from build123d import *

# Parameters (mm, degrees)
SKETCH1_R           = 50
BOSS_EXTRUDE1_DEPTH = 20
SKETCH2_W           = 20
SKETCH2_H           = 75
BOSS_EXTRUDE2_DEPTH = 65
SKETCH3_R           = 7.5
CUT_EXTRUDE1_DEPTH  = 65
FILLET1_R           = 37.5
SKETCH4_R           = 41.355609665
BOSS_EXTRUDE3_DEPTH = 35
SKETCH8_R           = 15
CUT_EXTRUDE2_DEPTH  = 20
SKETCH10_W          = 5
SKETCH10_H          = 8.446283525


with BuildPart() as part:
    # Sketch1 → Boss-Extrude1 (new body)
    with BuildSketch(Plane.XY):
        Circle(SKETCH1_R)
    extrude(amount=BOSS_EXTRUDE1_DEPTH)

    # Sketch2 → Boss-Extrude2 (add)
    with BuildSketch(Plane(origin=(0, 0, 0), x_dir=(-1, 0, 0), z_dir=(0, 0, -1))):
        Rectangle(SKETCH2_W, SKETCH2_H)
    extrude(amount=BOSS_EXTRUDE2_DEPTH)

    # Sketch3 → Cut-Extrude1 (cut)
    with BuildSketch(Plane(origin=(10, 0, 0), x_dir=(0, 0, -1), z_dir=(1, 0, 0))):
        with Locations((39.996807152, 0)):
            Circle(SKETCH3_R)
    extrude(amount=-CUT_EXTRUDE1_DEPTH, mode=Mode.SUBTRACT)

    # Fillet1
    fillet1_edges = [part.edges().sort_by_distance(p)[0] for p in [
        (0, -37.5, -65),
        (0, 37.5, -65),
    ]]
    fillet(fillet1_edges, radius=FILLET1_R - 0.0001)  # a hair under: the kernel refuses the full size

    # Sketch4 → Boss-Extrude3 (add)
    with BuildSketch(Plane.XY.offset(20)):
        Circle(SKETCH4_R)
    extrude(amount=BOSS_EXTRUDE3_DEPTH)

    # Sketch8 → Cut-Extrude2 (cut)
    with BuildSketch(Plane.XY.offset(55)):
        Circle(SKETCH8_R)
    extrude(amount=-CUT_EXTRUDE2_DEPTH, mode=Mode.SUBTRACT)

    # Sketch10 → Cut-Revolve1 (revolve, cut)
    with BuildSketch(Plane(origin=(0, 0, 0), x_dir=(0, 0, -1), z_dir=(1, 0, 0)), mode=Mode.PRIVATE) as cut_revolve1_sk:
        with Locations((-37.5, 15.776858238)):
            Rectangle(SKETCH10_W, SKETCH10_H)
    revolve(cut_revolve1_sk.sketch.rotate(Axis((0, 0, 55), (0, 0, -1)), 90), axis=Axis((0, 0, 55), (0, 0, -1)), mode=Mode.SUBTRACT)


solid = part.part
Geometry: final body of the model. Coordinates: model frame, mm. A direction names the side the tool comes from. Coordinates: 2 decimals unless noted, no trailing zeros. Loops run counter-clockwise (first coordinate to the right, second up) from the corner with the lowest first, then second, coordinate; pieces in that order, holes last. Notation, with made-up numbers: (45, -14) - (86, -14) arc R4 ccw to (86, -8) - close; hole circle Ø3 at (-34, -19.75). An arc over 180 degrees is marked (long way). Put each result on its own line as item: value. Start each with the question number.
Q1. Set-up query: faces 5 (the cylindrical face through (-14.985, 0.66, 47.605)), 6 (the flat face through (0, -37.5, -14)), 7 (the flat face through (0, 37.5, -14)), 8 (the flat face through (0, 0, 35)), 9 (the flat face through (10, -1, -32)). Return all of +Z, -Z, +X, -X, +Y, -Y with unobstructed straight access to the full face (end or side cutting, diameter ignored); none if empty.
Q2. Pull-direction query (Z, two-part tool) for faces 1 (the flat face through (-10, -1, -32)), 2 (the flat face through (-3, -15, 40)), 3 (the cylindrical face through (-0.14, -26.81, -53.72)), 4 (the flat face through (18, 1, 55)); classes: released by +Z, released by -Z, zero draft, split by the parting line, or undercut.
Q3. Line query: line 1 (Y direction, x = 0, z = 37); line 2 (Y direction, x = 0, z = 44); line 3 (Z direction, x = -17, y = -4.5). Output: solid intervals per line, ascending.
Q4. Pin query (flat end, axial travel): pin 1 Ø8 at (x, z) = (-11, 21) entering from +Y; pin 2 Ø19.5 at (y, z) = (0, -40) entering from -X; pin 3 Ø6 at (x, z) = (-2.5, -19.5) entering from +Y. Return the tip coordinate at first contact, or that it passes through.
Q5. Cut plane C-C, the plane y = 3. Return loops of the section in (x, z), and give its area (3 significant figures).
Q6. Cut plane D-D, the plane x = -33.5. Return loops of the section in (y, z).
Q7. Cut plane B-B, the plane z = 47. Return loops of the section in (x, y), and give its area (3 significant figures).
Filled sheet:
1. face 5: +Z
1. face 6: -Z, +X, -X, -Y
1. face 7: -Z, +X, -X, +Y
1. face 8: none
1. face 9: -Z, +X, +Y, -Y
2. face 1: zero draft
2. face 2: undercut
2. face 3: released by -Z
2. face 4: released by +Z
3. line 1: -41.36 to -20, 20 to 41.36
3. line 2: -41.36 to -15, 15 to 41.36
3. line 3: 0 to 35, 40 to 55
4. pin 1: y = 49.49
4. pin 2: x = -10
4. pin 3: y = 37.5
5. outline: (-49.91, 0) - (-10, 0) - (-10, -33.12) - (10, -33.12) - (10, 0) - (49.91, 0) - (49.91, 20) - (41.25, 20) - (41.25, 55) - (14.7, 55) - (14.7, 40) - (19.77, 40) - (19.77, 35) - (-19.77, 35) - (-19.77, 40) - (-14.7, 40) - (-14.7, 55) - (-41.25, 55) - (-41.25, 20) - (-49.91, 20) - close; (-10, -64.88) - (10, -64.88) - (10, -46.87) - (-10, -46.87) - close
5. area: 5,270 mm²
6. outline: (-37.12, 0) - (37.12, 0) - (37.12, 20) - (24.25, 20) - (24.25, 55) - (-24.25, 55) - (-24.25, 20) - (-37.12, 20) - close
7. outline: circle Ø82.71 at (0, 0); hole circle Ø30 at (0, 0)
7. area: 4,670 mm²
